Design review of the part built by this model. Coordinates are the model's own, in mm. Face numbers are marked on the shaded views. A direction names the side the tool comes from. Give positions to 0.01 mm unless a question says otherwise; leave off trailing zeros. Loops run counter-clockwise (first coordinate to the right, second up) from the corner with the lowest first, then second, coordinate; pieces in that order, holes last. Notation, with made-up numbers: M 25,0 L 80,0 A24 ccw 80,18 Z; hole C 84.25,58.5 d5. An arc over 180 degrees is marked long. Use a Markdown table: item, result. Add a question column.
(1) For the marked faces 1 and 2, list the 3-axis set-ups (+Z, -Z, +X, -X, +Y, -Y) from which the entire face can be reached by the end or side of a thin tool; tool diameter is ignored.
(2) Add section C-C, the plane z = 10. Give the boundary of the cut face in (x, y).
(3) Insertion check: pin 1 Ø12 at (x, z) = (34, 12) entering from -Y; pin 2 Ø6.5 at (y, z) = (-10, 10) entering from +X; pin 3 Ø8 at (y, z) = (11, 26) entering from -X; pin 4 Ø6 at (y, z) = (1, 7) entering from -X. Each pin has a flat end and moves straight along its axis. Give the tip position at first contact, or say it passes through.
(4) Add section D-D, the plane y = -15. Give the boundary of the cut face in (x, z).
(5) Add section A-A, the plane z = 35.5. Give the boundary of the cut face in (x, y), then the cut area to 3 significant figures.
(6) Draft analysis for pull direction X (two halves, no side actions). For the marked faces 3, 4, 5 and 6, state which applies: pulls with the +X half, pulls with the -X half, needs draft (parallel to the pull), parting line crosses it, or undercut.
(7) For probe 1 along Y at (x, z) = (111, 16); probe 2 along Y at (x, z) = (166, 10); probe 3 along X at (y, z) = (-15, 28), list the stretches that pass through material, from the lowest coordinate up.
(8) Add section B-B, the plane x = 98. Give the boundary of the cut face in (y, z).
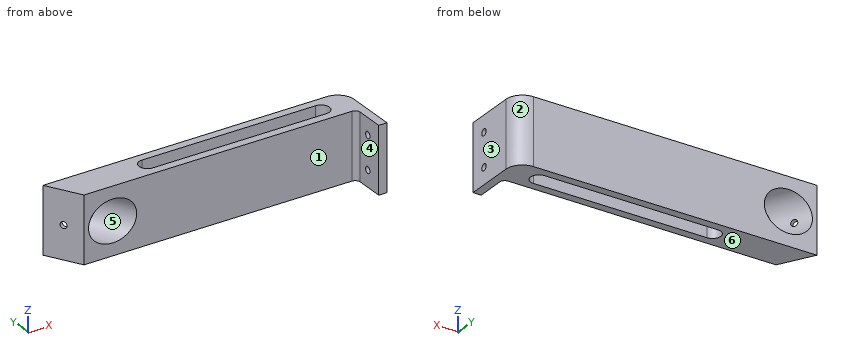
```python
from build123d import *

# Parameters (mm, degrees)
EXTRUDE_1_DEPTH          = 40
SKETCH_2_R               = 12.6
CUT_EXTRUDE_1_DEPTH      = 187.974102923
CUT_EXTRUDE_2_REACH      = 177.784
CUT_EXTRUDE_2_END_RADIUS = 12.6
SKETCH_3_R               = 2
SKETCH_4_W               = 5
SKETCH_4_H               = 40
EXTRUDE_2_DEPTH          = 20
SKETCH_5_R               = 2
CUT_EXTRUDE_3_DEPTH      = 183.123159192
FILLET_1_R               = 10
FILLET_2_R               = 3
CUT_EXTRUDE_4_DEPTH      = 176.783958324


with BuildPart() as part:
    # 草图1 → 凸台-拉伸1 (new body)
    with BuildSketch(Plane.XY):
        Polygon((0, 0), (170, 0), (170, 20), (-11.547005384, 20), align=None)
    extrude(amount=EXTRUDE_1_DEPTH)

    # 草图2 → 切除-拉伸1 (cut, through all)
    with BuildSketch(Plane(origin=(-11.547005384, 20, 0), x_dir=(0, 0, -1), z_dir=(-0.4999999999999949, 0.8660254037844416, 0))):
        with Locations(Location((-20, -15, 0), (0, 0, 90))):
            Circle(SKETCH_2_R)
    extrude(amount=-CUT_EXTRUDE_1_DEPTH, mode=Mode.SUBTRACT)

    # 切除-拉伸2: up to this cylinder (the profile starts outside it)
    cut_extrude_2_end = Plane(origin=(7.25676472, 17.430914806, 20), z_dir=(-0.4999999999999949, 0.8660254037844416, 0)) * Cylinder(CUT_EXTRUDE_2_END_RADIUS, 381.768, mode=Mode.PRIVATE)
    # 草图3 → 切除-拉伸2 (cut, up to the surface)
    with BuildSketch(Plane(origin=(0, 0, 0), x_dir=(0, 0, 1), z_dir=(-0.8660254037844417, -0.4999999999999949, 0)), mode=Mode.PRIVATE) as cut_extrude_2_sk1:
        with Locations(Location((20, 11.46723296, 0), (0, 0, 270))):
            Circle(SKETCH_3_R)
    cut_extrude_2_tool1 = extrude(cut_extrude_2_sk1.sketch, amount=-CUT_EXTRUDE_2_REACH, mode=Mode.PRIVATE) - cut_extrude_2_end
    add(cut_extrude_2_tool1.solids().sort_by_distance((-5.733616, 9.930915, 20))[0], mode=Mode.SUBTRACT)

    # 草图4 → 凸台-拉伸2 (add)
    with BuildSketch(Plane.XZ):
        with Locations((167.5, 20)):
            Rectangle(SKETCH_4_W, SKETCH_4_H)
    extrude(amount=EXTRUDE_2_DEPTH)

    # 草图5 → 切除-拉伸3 (cut, through all)
    with BuildSketch(Plane.ZY.offset(-165)):
        with Locations((10, -10)):
            Circle(SKETCH_5_R)
        with Locations(Location((30, -10, 0), (0, 0, 180))):
            Circle(SKETCH_5_R)
    extrude(amount=-CUT_EXTRUDE_3_DEPTH, mode=Mode.SUBTRACT)

    # 圆角1
    fillet_1_edges = [part.edges().sort_by_distance(p)[0] for p in [
        (170, 20, 20),
    ]]
    fillet(fillet_1_edges, radius=FILLET_1_R)

    # 圆角2
    fillet_2_edges = [part.edges().sort_by_distance(p)[0] for p in [
        (165, 0, 20),
    ]]
    fillet(fillet_2_edges, radius=FILLET_2_R)

    # 草图6 → 切除-拉伸4 (cut, through all)
    with BuildSketch(Plane(origin=(0, 0, 0), x_dir=(-1, 0, 0), z_dir=(0, 0, -1))):
        with BuildLine():
            Line((-150, 15), (-45, 15))
            ThreePointArc((-45, 15), (-40, 10), (-45, 5))
            Line((-45, 5), (-150, 5))
            ThreePointArc((-150, 5), (-155, 10), (-150, 15))
        make_face()
    extrude(amount=-CUT_EXTRUDE_4_DEPTH, mode=Mode.SUBTRACT)


solid = part.part
```
Established:
| question | item | result |
|---|---|---|
| 1 | face 1 | +Z, -Z, -X, -Y |
| 1 | face 2 | +Z, -Z, +X, +Y |
| 2 | outline | M -11.55,20 L 0,0 L 8.47,0 L -3.08,20 Z; M 14.62,20 L 26.17,0 L 162,0 A3 cw 165,-3 L 165,-8 L 170,-8 L 170,10 A10 ccw 160,20 Z; M 165,-20 L 170,-20 L 170,-12 L 165,-12 Z; hole M 45,5 L 150,5 A5 ccw 150,15 L 45,15 A5 ccw Z |
| 3 | pin 1 | y = 0 |
| 3 | pin 2 | x = 170 |
| 3 | pin 3 | x = -8.66 |
| 3 | pin 4 | x = -2.31 |
| 4 | outline | M 165,0 L 170,0 L 170,40 L 165,40 Z |
| 5 | outline | M -11.55,20 L 0,0 L 162,0 A3 cw 165,-3 L 165,-20 L 170,-20 L 170,10 A10 ccw 160,20 Z; hole M 45,5 L 150,5 A5 ccw 150,15 L 45,15 A5 ccw Z |
| 5 | area | 2,470 mm^2 |
| 6 | face 3 | pulls with the +X half |
| 6 | face 4 | pulls with the -X half |
| 6 | face 5 | undercut |
| 6 | face 6 | needs draft |
| 7 | probe 1 | 0 to 5, 15 to 20 |
| 7 | probe 2 | -20 to -12, -8 to 18 |
| 7 | probe 3 | 165 to 170 |
| 8 | outline | M 0,0 L 5,0 L 5,40 L 0,40 Z; M 15,0 L 20,0 L 20,40 L 15,40 Z |
